Here's how the part is built. I have some questions about the finished solid (model axes, mm). Face numbers are marked on the shaded views. Coordinates: 2 decimals unless noted, no trailing zeros. Write each loop counter-clockwise with the first axis right and the second up, starting at its lowest first coordinate (ties: lowest second). Pieces come first, ordered by that corner, then holes. Notation, with made-up numbers: (-18, 88) -> (40, 88) arc R27 ccw to (40, 105) -> close; hole circle Ø10 at (23, -15.75). An arc over 180 degrees is marked (long way). Use a Markdown table: item, result. Add a question column.
Item 1: Imagine slicing it at A-A, the plane z = 2.75. Write out the boundary of the cut face in (x, y), and give its area (3 significant figures).
Item 2: If we mould it in two halves opening along X, with no side actions, what happens to the marked faces 1, 2 and 3? For each: pulls with the +X half, pulls with the -X half, needs draft (parallel to the pull), parting line crosses it, or undercut.
Item 3: Will these pins go through, and if not, where does the flat tip stop? pin 1 Ø1.5 at (x, y) = (-6.5, 13.5) entering from -Z; pin 2 Ø2 at (y, z) = (59.5, 2) entering from -X; pin 3 Ø3.5 at (x, z) = (-7.5, -0.5) entering from -Y.
Item 4: Imagine slicing it at B-B, the plane y = 17. Write out the boundary of the cut face in (x, z).
Item 5: Imagine slicing it at D-D, the plane x = 16. Write out the boundary of the cut face in (y, z), and give its area (3 significant figures).
Item 6: Imagine slicing it at C-C, the plane y = 50. Write out the boundary of the cut face in (x, z).
Item 7: If I drill on line 1 along Z through (x, y) = (25, 42.5); line 2 along X through (y, z) = (55, 3); line 3 along Y through (x, z) = (3, -1), over which ranges is the centre line in solid material (lowest first)? Write a range as from..to.
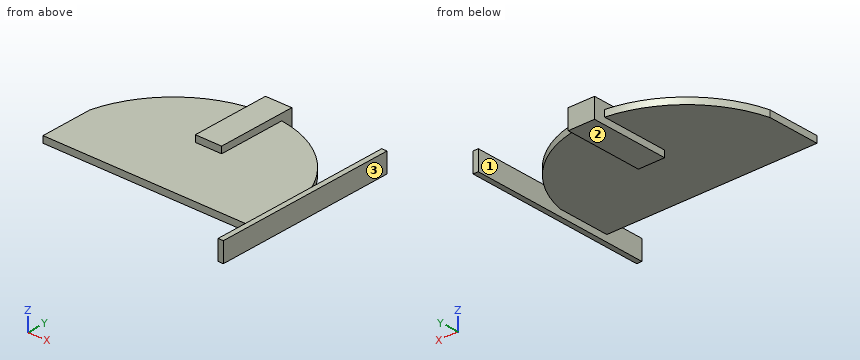
```python
from build123d import *

# Parameters (mm, degrees)
F1_DEPTH = 1.5875
F2_DEPTH = 1.5875
F3_DEPTH = 4.7625
F4_DEPTH = 4.7625
F5_W     = 19.05
F5_H     = 3.175
F5_W_2   = 25.4
F5_W_3   = 44.45
F6_DEPTH = 2.54


with BuildPart() as f1:
    # F0 (on Top) → F1 (new body)
    with BuildSketch(Plane.XY):
        with BuildLine():
            Line((-50.8, 0), (0, 0))
            Line((0, 0), (50.8, 0))
            Line((50.8, 0), (50.8, 25.4))
            ThreePointArc((50.8, 25.4), (34.8924839126, 52.4357961473), (6.35, 65.4477119742))
            Line((6.35, 65.4477119742), (6.35, 32.8159203153))
            Line((6.35, 32.8159203153), (0, 32.8159203153))
            Line((0, 32.8159203153), (-6.35, 32.8159203153))
            Line((-6.35, 32.8159203153), (-6.35, 65.4477119742))
            ThreePointArc((-6.35, 65.4477119742), (-34.8924839126, 52.4357961473), (-50.8, 25.4))
            Line((-50.8, 25.4), (-50.8, 0))
        make_face()
    extrude(amount=F1_DEPTH)

    # F2 (add): a face of the model
    f2_faces = [f1.faces().sort_by_distance(p)[0] for p in [
        (0, 27.1005445022, 0),
    ]]
    extrude(f2_faces, amount=F2_DEPTH)

    # F0 (on Top) → F3 (join)
    with BuildSketch(Plane.XY):
        with BuildLine():
            ThreePointArc((6.35, 65.4477119742), (0, 65.8359203153), (-6.35, 65.4477119742))
            Line((-6.35, 65.4477119742), (-6.35, 32.8159203153))
            Line((-6.35, 32.8159203153), (0, 32.8159203153))
            Line((0, 32.8159203153), (6.35, 32.8159203153))
            Line((6.35, 32.8159203153), (6.35, 65.4477119742))
        make_face()
        with BuildLine():
            Line((-6.35, 70.9159203153), (-6.35, 65.4477119742))
            ThreePointArc((-6.35, 65.4477119742), (0, 65.8359203153), (6.35, 65.4477119742))
            Line((6.35, 65.4477119742), (6.35, 70.9159203153))
            Line((6.35, 70.9159203153), (0, 70.9159203153))
            Line((0, 70.9159203153), (-6.35, 70.9159203153))
        make_face()
    extrude(amount=F3_DEPTH)

    # F0 (on Top) → F4 (join)
    with BuildSketch(Plane.XY):
        with BuildLine():
            ThreePointArc((6.35, 65.4477119742), (0, 65.8359203153), (-6.35, 65.4477119742))
            Line((-6.35, 65.4477119742), (-6.35, 32.8159203153))
            Line((-6.35, 32.8159203153), (0, 32.8159203153))
            Line((0, 32.8159203153), (6.35, 32.8159203153))
            Line((6.35, 32.8159203153), (6.35, 65.4477119742))
        make_face()
        with BuildLine():
            Line((-6.35, 70.9159203153), (-6.35, 65.4477119742))
            ThreePointArc((-6.35, 65.4477119742), (0, 65.8359203153), (6.35, 65.4477119742))
            Line((6.35, 65.4477119742), (6.35, 70.9159203153))
            Line((6.35, 70.9159203153), (0, 70.9159203153))
            Line((0, 70.9159203153), (-6.35, 70.9159203153))
        make_face()
    extrude(amount=-F4_DEPTH)

    # F5 (on face) → F6 (join)
    with BuildSketch(Plane.YZ.offset(50.8)):
        with Locations((-9.525, 0)):
            Rectangle(F5_W, F5_H)
        Polygon((-19.05, 1.5875), (0, 1.5875), (25.4, 1.5875), (69.85, 1.5875), (69.85, 4.7625), (-19.05, 4.7625), align=None)
        with Locations((12.7, 0)):
            Rectangle(F5_W_2, F5_H)
        with Locations((47.625, 0)):
            Rectangle(F5_W_3, F5_H)
        Polygon((25.4, -1.5875), (0, -1.5875), (-19.05, -1.5875), (-19.05, -4.7625), (69.85, -4.7625), (69.85, -1.5875), align=None)
    extrude(amount=F6_DEPTH)


solid = f1.part
```
Ans:
| question | item | result |
|---|---|---|
| 1 | outline | (-6.35, 32.82) -> (6.35, 32.82) -> (6.35, 70.92) -> (-6.35, 70.92) -> close; (50.8, -19.05) -> (53.34, -19.05) -> (53.34, 69.85) -> (50.8, 69.85) -> close |
| 1 | area | 710 mm^2 |
| 2 | face 1 | undercut |
| 2 | face 2 | needs draft |
| 2 | face 3 | pulls with the +X half |
| 3 | pin 1 | stops at z = -1.59 |
| 3 | pin 2 | stops at x = -26.51 |
| 3 | pin 3 | stops at y = 0 |
| 4 | outline | (-50.8, -1.59) -> (50.8, -1.59) -> (50.8, -4.76) -> (53.34, -4.76) -> (53.34, 4.76) -> (50.8, 4.76) -> (50.8, 1.59) -> (-50.8, 1.59) -> close |
| 5 | outline | (0, -1.59) -> (63.32, -1.59) -> (63.32, 1.59) -> (0, 1.59) -> close |
| 5 | area | 201 mm^2 |
| 6 | outline | (-37.42, -1.59) -> (-6.35, -1.59) -> (-6.35, -4.76) -> (6.35, -4.76) -> (6.35, -1.59) -> (37.42, -1.59) -> (37.42, 1.59) -> (6.35, 1.59) -> (6.35, 4.76) -> (-6.35, 4.76) -> (-6.35, 1.59) -> (-37.42, 1.59) -> close; (50.8, -4.76) -> (53.34, -4.76) -> (53.34, 4.76) -> (50.8, 4.76) -> close |
| 7 | line 1 | z = -1.59..1.59 |
| 7 | line 2 | x = -6.35..6.35, 50.8..53.34 |
| 7 | line 3 | y = 0..70.92 |
